Print and shaded views of the part. All mm, measured from the part's lowest x, y and z. Coordinates: 2 decimals unless noted, no trailing zeros. Order: outer loops, then holes, each group sorted by start corner. A loop starts at its lowest first (then second) coordinate and runs counter-clockwise, first axis right, second up. Notation, with made-up numbers: M -37.5,67.5 L 19.5,67.5 A16 ccw 19.5,85.5 Z; hole C 71.25,-15 d7. An arc over 180 degrees is marked long. Return JSON: item names as keys, results as strings.
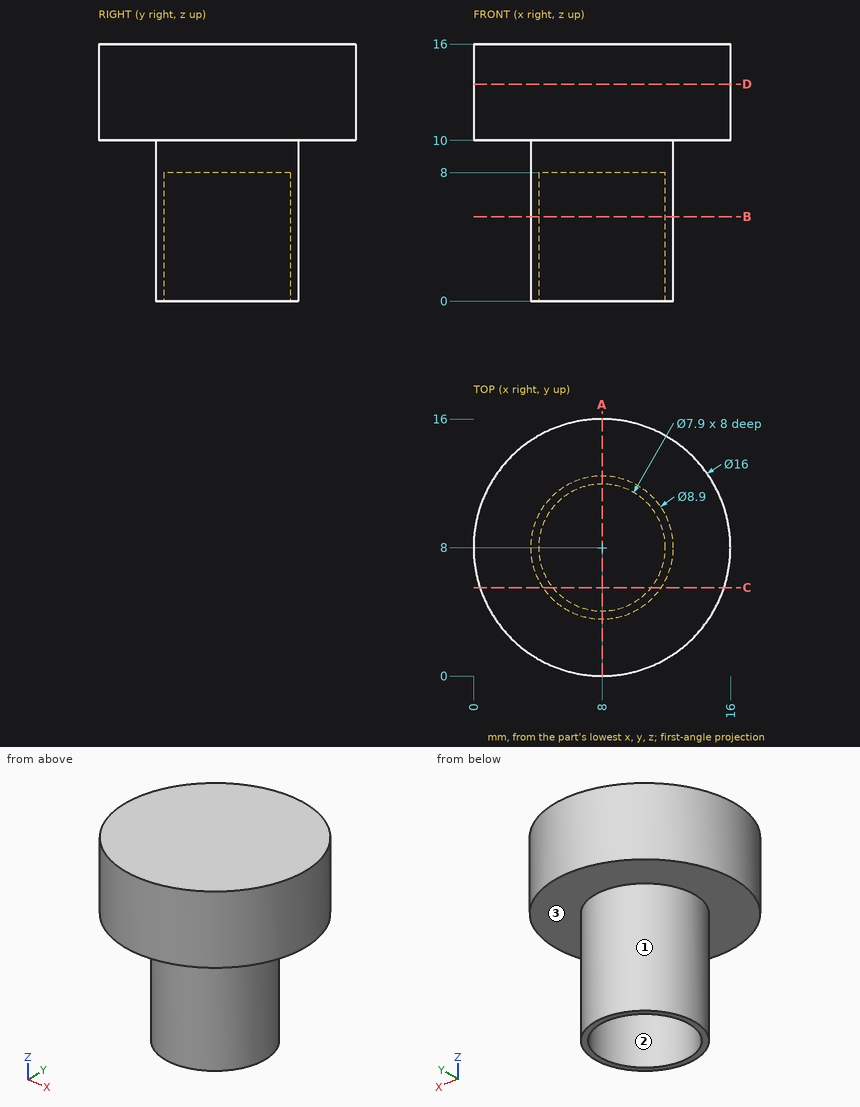
Item 1: Pull direction Y, two halves, no side cores. Call the marked faces 1, 2 and 3: +Y half, -Y half, draft (parallel to the pull), parting line (faces both ways), or undercut.
Check result:
{"face 1": "parting line", "face 2": "undercut", "face 3": "draft"}
Item 2: Saw through at A-A (x = 8). Write the cut outline in (y, z).
Check result:
{"outline": "M 0,10 L 3.55,10 L 3.55,0 L 4.05,0 L 4.05,8 L 11.95,8 L 11.95,0 L 12.45,0 L 12.45,10 L 16,10 L 16,16 L 0,16 Z"}
Item 3: Saw through at B-B (z = 5.25). Write the cut outline in (x, y).
Check result:
{"outline": "C 8,8 d8.9; hole C 8,8 d7.9"}
Item 4: Saw through at D-D (z = 13.5). Write the cut outline in (x, y), and give its area (3 significant figures).
Check result:
{"outline": "C 8,8 d16", "area": "201 mm2"}
Item 5: Drop flat-ended pins along their axis: pin 1 Ø5 at (x, y) = (11, 6.5) entering from -Z; pin 2 Ø2.5 at (x, y) = (8.5, 8.5) entering from -Z; pin 3 Ø1 at (y, z) = (8, 3.5) entering from +X; pin 4 Ø1 at (x, z) = (4.5, 14) entering from +Y. Give the stop position or say it passes through.
Check result:
{"pin 1": "stops at z = 0", "pin 2": "stops at z = 8", "pin 3": "stops at x = 12.45", "pin 4": "stops at y = 15.42"}
Item 6: Wall check: line 1 (Y direction, x = 8, z = 2.75); line 2 (X direction, y = 11, z = 4.75); line 3 (Z direction, x = 14, y = 10). Give the ranges that are in metal, low to high.
Check result:
{"line 1": "y = 3.55 to 4.05, 11.95 to 12.45", "line 2": "x = 4.71 to 5.43, 10.57 to 11.29", "line 3": "z = 10 to 16"}
Item 7: Saw through at C-C (y = 5.5). Write the cut outline in (x, z).
Check result:
{"outline": "M 0.4,10 L 4.32,10 L 4.32,0 L 4.94,0 L 4.94,8 L 11.06,8 L 11.06,0 L 11.68,0 L 11.68,10 L 15.6,10 L 15.6,16 L 0.4,16 Z"}
